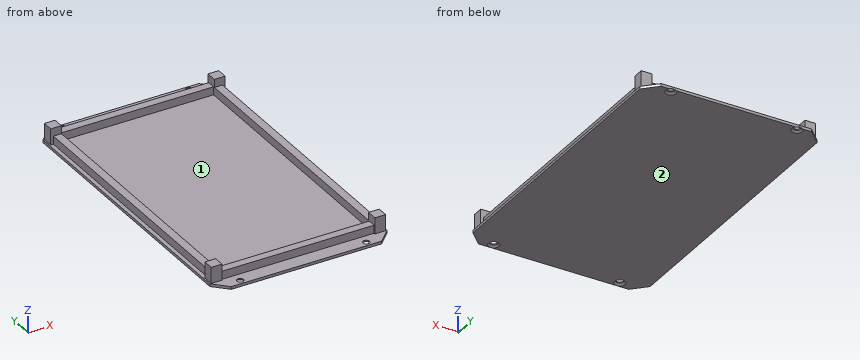
from build123d import *

# Parameters (mm, degrees)
BOX022_W          = 63
BOX022_H          = 3
BOX022_DEPTH      = 3
BOX023_W          = 3
BOX023_H          = 104
BOX023_DEPTH      = 3
BOX024_W          = 3
BOX024_H          = 104
BOX024_DEPTH      = 3
BOX018_W          = 4
BOX018_H          = 4
BOX018_DEPTH      = 6
BOX017_W          = 4
BOX017_H          = 4
BOX017_DEPTH      = 6
BOX020_W          = 4
BOX020_H          = 4
BOX020_DEPTH      = 6
BOX019_W          = 4
BOX019_H          = 4
BOX019_DEPTH      = 6
BOX021_W          = 63
BOX021_H          = 3
BOX021_DEPTH      = 3
CYLINDER001_R     = 1.2
CYLINDER001_DEPTH = 1
CYLINDER002_R     = 1.2
CYLINDER002_DEPTH = 1
CYLINDER003_R     = 1.2
CYLINDER003_DEPTH = 1
CYLINDER_R        = 1.2
CYLINDER_DEPTH    = 1
PAD003_DEPTH      = 1


with BuildPart() as cone002:
    # Cone002 → Cone002 (revolve)
    with BuildSketch(Plane(origin=(10, 109, -16.5), x_dir=(1, 0, 0), z_dir=(0, 1, 0))):
        Polygon((0, 0), (2, 1.5), (0, 1.5), align=None)
    revolve(axis=Axis((10, 109, -16.5), (0, 0, -1)))


with BuildPart() as cone001:
    # Cone001 → Cone001 (revolve)
    with BuildSketch(Plane(origin=(10, -2.5, -16.5), x_dir=(1, 0, 0), z_dir=(0, 1, 0))):
        Polygon((0, 0), (2, 1.5), (0, 1.5), align=None)
    revolve(axis=Axis((10, -2.5, -16.5), (0, 0, -1)))


with BuildPart() as cone003:
    # Cone003 → Cone003 (revolve)
    with BuildSketch(Plane(origin=(57, 109, -16.5), x_dir=(1, 0, 0), z_dir=(0, 1, 0))):
        Polygon((0, 0), (2, 1.5), (0, 1.5), align=None)
    revolve(axis=Axis((57, 109, -16.5), (0, 0, -1)))


with BuildPart() as fusion010:
    # Cone → Cone (revolve)
    with BuildSketch(Plane(origin=(57, -2.5, -16.5), x_dir=(1, 0, 0), z_dir=(0, 1, 0))):
        Polygon((0, 0), (2, 1.5), (0, 1.5), align=None)
    revolve(axis=Axis((57, -2.5, -16.5), (0, 0, -1)))

    # Fusion010: union Cone002, Cone001, Cone003
    add(cone002.part)
    add(cone001.part)
    add(cone003.part)


with BuildPart() as cube022:
    # Box022 → Box022 (new body)
    with BuildSketch(Plane(origin=(2, 102, -17), x_dir=(1, 0, 0), z_dir=(0, 0, 1))):
        with Locations((31.5, 1.5)):
            Rectangle(BOX022_W, BOX022_H)
    extrude(amount=BOX022_DEPTH)


with BuildPart() as cube023:
    # Box023 → Box023 (new body)
    with BuildSketch(Plane(origin=(2, 1, -17), x_dir=(1, 0, 0), z_dir=(0, 0, 1))):
        with Locations((1.5, 52)):
            Rectangle(BOX023_W, BOX023_H)
    extrude(amount=BOX023_DEPTH)


with BuildPart() as cube024:
    # Box024 → Box024 (new body)
    with BuildSketch(Plane(origin=(62, 1, -17), x_dir=(1, 0, 0), z_dir=(0, 0, 1))):
        with Locations((1.5, 52)):
            Rectangle(BOX024_W, BOX024_H)
    extrude(amount=BOX024_DEPTH)


with BuildPart() as cube018:
    # Box018 → Box018 (new body)
    with BuildSketch(Plane(origin=(1, 101.5, -17), x_dir=(1, 0, 0), z_dir=(0, 0, 1))):
        with Locations((2, 2)):
            Rectangle(BOX018_W, BOX018_H)
    extrude(amount=BOX018_DEPTH)


with BuildPart() as cube017:
    # Box017 → Box017 (new body)
    with BuildSketch(Plane(origin=(1, 0.5, -17), x_dir=(1, 0, 0), z_dir=(0, 0, 1))):
        with Locations((2, 2)):
            Rectangle(BOX017_W, BOX017_H)
    extrude(amount=BOX017_DEPTH)


with BuildPart() as cube020:
    # Box020 → Box020 (new body)
    with BuildSketch(Plane(origin=(62, 0.5, -17), x_dir=(1, 0, 0), z_dir=(0, 0, 1))):
        with Locations((2, 2)):
            Rectangle(BOX020_W, BOX020_H)
    extrude(amount=BOX020_DEPTH)


with BuildPart() as cube019:
    # Box019 → Box019 (new body)
    with BuildSketch(Plane(origin=(62, 101.5, -17), x_dir=(1, 0, 0), z_dir=(0, 0, 1))):
        with Locations((2, 2)):
            Rectangle(BOX019_W, BOX019_H)
    extrude(amount=BOX019_DEPTH)


with BuildPart() as fusion011:
    # Box021 → Box021 (new body)
    with BuildSketch(Plane(origin=(2, 1, -17), x_dir=(1, 0, 0), z_dir=(0, 0, 1))):
        with Locations((31.5, 1.5)):
            Rectangle(BOX021_W, BOX021_H)
    extrude(amount=BOX021_DEPTH)

    # Fusion011: union Cube022, Cube023, Cube024, Cube018, Cube017, Cube020, Cube019
    add(cube022.part)
    add(cube023.part)
    add(cube024.part)
    add(cube018.part)
    add(cube017.part)
    add(cube020.part)
    add(cube019.part)


with BuildPart() as cylinder001:
    # Cylinder001 → Cylinder001 (new body)
    with BuildSketch(Plane(origin=(57, -2.5, -18), x_dir=(1, 0, 0), z_dir=(0, 0, 1))):
        Circle(CYLINDER001_R)
    extrude(amount=CYLINDER001_DEPTH)


with BuildPart() as cylinder002:
    # Cylinder002 → Cylinder002 (new body)
    with BuildSketch(Plane(origin=(57, 109, -18), x_dir=(1, 0, 0), z_dir=(0, 0, 1))):
        Circle(CYLINDER002_R)
    extrude(amount=CYLINDER002_DEPTH)


with BuildPart() as cylinder003:
    # Cylinder003 → Cylinder003 (new body)
    with BuildSketch(Plane(origin=(10, 109, -18), x_dir=(1, 0, 0), z_dir=(0, 0, 1))):
        Circle(CYLINDER003_R)
    extrude(amount=CYLINDER003_DEPTH)


with BuildPart() as fusion006:
    # Cylinder → Cylinder (new body)
    with BuildSketch(Plane(origin=(10, -2.5, -18), x_dir=(1, 0, 0), z_dir=(0, 0, 1))):
        Circle(CYLINDER_R)
    extrude(amount=CYLINDER_DEPTH)

    # Fusion006: union Cylinder001, Cylinder002, Cylinder003
    add(cylinder001.part)
    add(cylinder002.part)
    add(cylinder003.part)


with BuildPart() as cut004:
    # Sketch003 → Pad003 (new body)
    with BuildSketch(Plane.XY.offset(-18)):
        Polygon((0.5, 0.5), (5.5, -4.5), (61.5, -4.5), (66.5, 0.5), (66.5, 105.5), (61.5, 110.5), (5.5, 110.5), (0.5, 105.5), align=None)
    extrude(amount=PAD003_DEPTH)

    # Cut002: cut Fusion006
    add(fusion006.part, mode=Mode.SUBTRACT)

    # Fusion012: union Fusion011
    add(fusion011.part)

    # Cut004: cut Fusion010
    add(fusion010.part, mode=Mode.SUBTRACT)


solid = cut004.part
The listing builds one solid part. Answer for the finished solid, in the listing's coordinates (mm). Face numbers are marked on the shaded views. Round coordinates to 2 decimals unless told otherwise and drop trailing zeros. Write each loop counter-clockwise with the first axis right and the second up, starting at its lowest first coordinate (ties: lowest second). Pieces come first, ordered by that corner, then holes. Notation, with made-up numbers: (37, 89.5) - (73, 89.5) arc R25 cw to (73, 114.5) - close; hole circle Ø3 at (80.25, -1.5). An arc over 180 degrees is marked (long way). Use one line per item in the form item = value. Start each with the question number.
Item 1: Determine the mould class of the marked faces 1 and 2 for opening direction Y: +Y half, -Y half, draft (parallel to the pull), parting line (faces both ways), or undercut.
Item 2: A cutting plane is placed at B-B (x = 16). Write down the section's boundary in (y, z).
Item 3: A cutting plane is placed at A-A (y = -2.5). Write down the section's boundary in (x, z), plus the area to 3 significant figures.
Item 4: Flat-ended cylindrical pins translate along their axes: pin 1 Ø0.9 at (x, y) = (3.5, 76) entering from +Z; pin 2 Ø3 at (x, z) = (35, -16.5) entering from -Y; pin 3 Ø1 at (x, y) = (49, 79) entering from +Z; pin 4 Ø2 at (x, y) = (57, 109) entering from -Z. Find the tip coordinate at first contact, or state that the pin passes through.
Item 5: Find the intervals of material crossed by line 1 (Y direction, x = 10, z = -17.2); line 2 (Y direction, x = 14, z = -14.75); line 3 (X direction, y = 109, z = -17.2), in increasing order. Write a range as [from, to].
Item 6: A cutting plane is placed at C-C (y = 83). Write down the section's boundary in (x, z), plus the area to 3 significant figures.
The answers:
q1.face_1 = undercut
q1.face_2 = draft
q2.outline = (-4.5, -18) - (110.5, -18) - (110.5, -17) - (105, -17) - (105, -14) - (102, -14) - (102, -17) - (4, -17) - (4, -14) - (1, -14) - (1, -17) - (-4.5, -17) - close
q3.outline = (3.5, -18) - (8, -18) - (8.8, -17.4) - (8.8, -17) - (3.5, -17) - close; (11.2, -17.4) - (12, -18) - (55, -18) - (55.8, -17.4) - (55.8, -17) - (11.2, -17) - close; (58.2, -17.4) - (59, -18) - (63.5, -18) - (63.5, -17) - (58.2, -17) - close
q3.area = 54.2 mm^2
q4.pin_1 = -14
q4.pin_2 = -4.5
q4.pin_3 = -17
q4.pin_4 = through
q5.line_1 = [-4.5, -3.7], [-1.3, 107.8], [110.2, 110.5]
q5.line_2 = [1, 4], [102, 105]
q5.line_3 = [4, 8.8], [11.2, 55.8], [58.2, 63]
q6.outline = (0.5, -18) - (66.5, -18) - (66.5, -17) - (65, -17) - (65, -14) - (62, -14) - (62, -17) - (5, -17) - (5, -14) - (2, -14) - (2, -17) - (0.5, -17) - close
q6.area = 84.0 mm^2
